from build123d import *

# Parameters (mm, degrees)
EXTRUDE_1_DEPTH          = 300
CUT_EXTRUDE_1_DEPTH      = 688.477272352
CUT_EXTRUDE_1_DEPTH_BACK = 688.477272352
SKETCH_3_W               = 560
SKETCH_3_H               = 150
CUT_EXTRUDE_2_DEPTH      = 470.041575982
EXTRUDE_2_DEPTH          = 50
FILLET_1_R               = 10
CUT_EXTRUDE_3_DEPTH      = 476.631159618
CUT_EXTRUDE_3_DEPTH_BACK = 476.631159618
SKETCH_5_R               = 10


with BuildPart() as part:
    # Эскиз1 → Бобышка-Вытянуть1 (new body)
    with BuildSketch(Plane.XY):
        Polygon((-300, -15), (-300, 0), (-300, 215), (-280, 215), (-280, 15), (280, 15), (280, 215), (300, 215), (300, 0), (300, -15), align=None)
    extrude(amount=EXTRUDE_1_DEPTH)

    # Эскиз2 → Вырез-Вытянуть1 (cut, two sides: drawn at the far end of the back side and taken through both)
    with BuildSketch(Plane(origin=(-280, 0, 0), x_dir=(0, 0, -1), z_dir=(1, 0, 0)).offset(-CUT_EXTRUDE_1_DEPTH_BACK)):
        Polygon((-150, 215), (0, 15), (0, 215), align=None)
    extrude(amount=CUT_EXTRUDE_1_DEPTH + CUT_EXTRUDE_1_DEPTH_BACK, mode=Mode.SUBTRACT)

    # Эскиз3 → Вырез-Вытянуть2 (cut, through all)
    with BuildSketch(Plane(origin=(0, 15, 0), x_dir=(1, 0, 0), z_dir=(0, 1, 0))):
        with Locations((0, -75)):
            Rectangle(SKETCH_3_W, SKETCH_3_H)
    extrude(amount=-CUT_EXTRUDE_2_DEPTH, mode=Mode.SUBTRACT)

    # Эскиз4 → Бобышка-Вытянуть2 (add)
    with BuildSketch(Plane.XZ.offset(15)):
        Polygon((-220, 300), (-300, 300), (-300, 150), (-280, 150), (-220, 150), align=None)
        Polygon((300, 300), (220, 300), (220, 150), (280, 150), (300, 150), align=None)
    extrude(amount=EXTRUDE_2_DEPTH)

    # Скругление1
    fillet_1_edges = [part.edges().sort_by_distance(p)[0] for p in [
        (0, -15, 150),
        (-220, -65, 225),
        (-220, -40, 150),
        (-220, -40, 300),
        (-260, -65, 150),
        (-260, -65, 300),
        (-300, -65, 225),
        (-220, -15, 225),
        (0, -15, 300),
        (220, -15, 225),
        (220, -40, 300),
        (220, -40, 150),
        (260, -65, 300),
        (220, -65, 225),
        (260, -65, 150),
        (300, -65, 225),
    ]]
    fillet(fillet_1_edges, radius=FILLET_1_R)

    # Эскиз5 → Вырез-Вытянуть3 (cut, two sides: drawn at the far end of the back side and taken through both)
    with BuildSketch(Plane.XY.offset(300).offset(-CUT_EXTRUDE_3_DEPTH_BACK)):
        with Locations((-260, -40)):
            Circle(SKETCH_5_R)
        with Locations((260, -40)):
            Circle(SKETCH_5_R)
    extrude(amount=CUT_EXTRUDE_3_DEPTH + CUT_EXTRUDE_3_DEPTH_BACK, mode=Mode.SUBTRACT)


solid = part.part
Input: part model. Units: mm. Frame: model coordinates. A direction names the side the tool comes from. Give positions to 0.01 mm unless a question says otherwise; leave off trailing zeros. Loops run counter-clockwise (first coordinate to the right, second up) from the corner with the lowest first, then second, coordinate; pieces in that order, holes last. Notation, with made-up numbers: (33.5, 48.25) - (64.5, 48.25) arc R7 ccw to (64.5, 55.25) - close; hole circle Ø11 at (3.5, -37.5). An arc over 180 degrees is marked (long way). Use CSV: the item, a comma, the result in double quotes. Start each with the question number.
Item 1: Section B-B on z = 81. Return loops of the section in (x, y), then the cut area to 3 significant figures.
Item 2: Line query: line 1 (X direction, y = -40, z = 210); line 2 (Y direction, x = -260, z = 224); line 3 (X direction, y = 25, z = 267.5). Output: solid intervals per line, ascending.
Item 3: Reachability of faces 1 (the flat face through (290, -15, 74)), 2 (the cylindrical face through (-250.763, -43.83, 223.95)), 3 (the flat face through (-4, 15, 224)), 4 (the flat face through (220, -40, 226)) from +Z, -Z, +X, -X, +Y, -Y: full face, straight path, thin tool, end or side. Return the list, or none.
Item 4: Contact query for flat-ended pins moving along their axis: P1, Ø16, axis at x = -260, y = -40, coming from the +Z side; P2, Ø4, axis at x = -50.5, z = 182, coming from the -Y side; P3, Ø3, axis at x = 101.5, z = 231.5, coming from the +Y side. Output: stop coordinate, or through.
Item 5: Section D-D on z = 230. Return loops of the section in (x, y).
Item 6: Section C-C on y = -40. Return loops of the section in (x, z), then the cut area to 3 significant figures.
Item 7: Section A-A on x = -260. Return loops of the section in (y, z), then the cut area to 3 significant figures.
Item 8: Mould query, pull axis X, two halves, no side actions, for faces 5 (the flat face through (-290, -15, 74)), 6 (the flat face through (-300, 82, 185)), 7 (the flat face through (-4, -4, 150)). Classes: pulls with the +X half, pulls with the -X half, needs draft (parallel to the pull), parting line crosses it, or undercut.
Ans:
1,outline,"(-300, -15) - (-280, -15) - (-280, 123) - (-300, 123) - close; (280, -15) - (300, -15) - (300, 123) - (280, 123) - close"
1,area,"5,520 mm2"
2,line 1,"x = -300 to -270, -250 to -220, 220 to 250, 270 to 300"
2,line 2,"y = -65 to -50, -30 to 15"
2,line 3,"x = -300 to -280, 280 to 300"
3,face 1,"-Z, +X, -X, -Y"
3,face 2,"+Z, -Z"
3,face 3,"+Z, -Z, +Y"
3,face 4,"+Z, -Z, -Y"
4,P1,"passes through"
4,P2,"stops at y = -15"
4,P3,"stops at y = 15"
5,outline,"(-300, -55) arc R10 ccw to (-290, -65) - (-230, -65) arc R10 ccw to (-220, -55) - (-220, -25) arc R10 cw to (-210, -15) - (210, -15) arc R10 cw to (220, -25) - (220, -55) arc R10 ccw to (230, -65) - (290, -65) arc R10 ccw to (300, -55) - (300, 215) - (280, 215) - (280, 15) - (-280, 15) - (-280, 215) - (-300, 215) - close; hole circle Ø20 at (-260, -40); hole circle Ø20 at (260, -40)"
6,outline,"(-300, 150) - (-270, 150) - (-270, 300) - (-300, 300) - close; (-250, 150) - (-230, 150) arc R10 ccw to (-220, 160) - (-220, 290) arc R10 ccw to (-230, 300) - (-250, 300) - close; (220, 160) arc R10 ccw to (230, 150) - (250, 150) - (250, 300) - (230, 300) arc R10 ccw to (220, 290) - close; (270, 150) - (300, 150) - (300, 300) - (270, 300) - close"
6,area,"17,900 mm2"
7,outline,"(-65, 160) arc R10 ccw to (-55, 150) - (-50, 150) - (-50, 300) - (-55, 300) arc R10 ccw to (-65, 290) - close; (-30, 150) - (15, 150) - (15, 300) - (-30, 300) - close"
7,area,"8,960 mm2"
8,face 5,"needs draft"
8,face 6,"pulls with the -X half"
8,face 7,"undercut"
